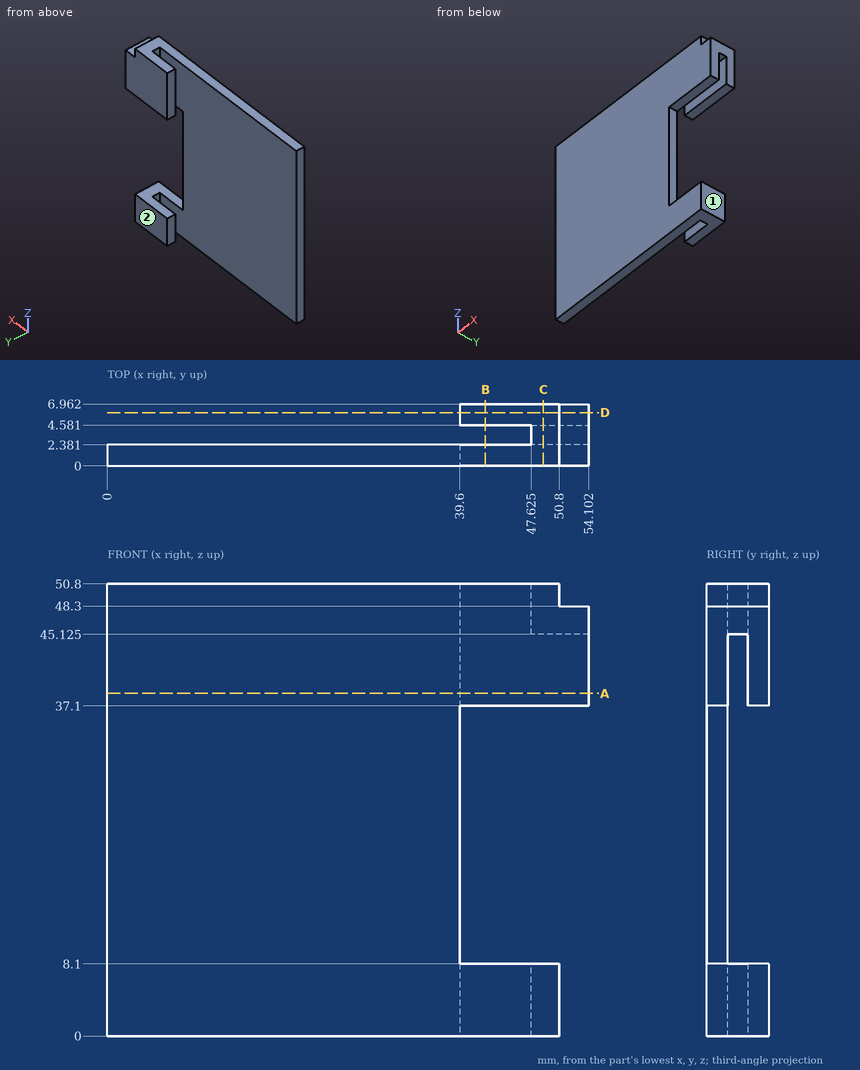
Could you check a few things on this drawing? It's one solid part, dimensions in mm from its lowest x, y, z. A direction names the side the tool comes from. Coordinates: 2 decimals unless noted, no trailing zeros. Write each loop counter-clockwise with the first axis right and the second up, starting at its lowest first coordinate (ties: lowest second). Pieces come first, ordered by that corner, then holes. Notation, with made-up numbers: (60.25, -26.5) - (106.25, -26.5) arc R24 ccw to (106.25, -9.5) - close; hole circle Ø7 at (-16.5, 6). An arc over 180 degrees is marked (long way). Return JSON: item names as keys, results as strings. Group by question number.
Item 1: If we section it at D-D (y = 6): Write out the boundary of the cut face in (x, z), then the cut area to 3 significant figures.
Item 2: If we section it at A-A (z = 38.5): Write out the boundary of the cut face in (x, y).
Item 3: I'm going to push flat-ended pins straight in: pin 1 Ø1.2 at (y, z) = (5.5, 3.5) entering from -X; pin 2 Ø1.2 at (x, y) = (46.5, 1.5) entering from -Z; pin 3 Ø1.1 at (y, z) = (3.5, 4.5) entering from -X (1 decimal); pin 4 Ø1.3 at (y, z) = (2.5, 50) entering from +X. Where does each tip first touch, or does it pass through?
Item 4: If we section it at B-B (x = 42.5): Write out the boundary of the cut face in (y, z), then the cut area to 3 significant figures.
Item 5: If we section it at C-C (x = 49): Write out the boundary of the cut face in (y, z) (1 decimal), then the cut area to 3 significant figures.
Item 6: Which directions (+Z, -Z, +X, -X, +Y, -Y) give clear straight access to the entire face, cutting with the end or side of a thin tool? Please do the marked faces 1 and 2.
Item 7: Please list where these lines run through material, in increasing order: probe 1 along Y at (x, z) = (36.5, 30.5); probe 2 along Z at (x, y) = (43.5, 6.75); probe 3 along Y at (x, z) = (40, 39.5).
Return value:
{
 "1": {"outline": "(39.6, 0) - (50.8, 0) - (50.8, 8.1) - (39.6, 8.1) - close; (39.6, 37.1) - (54.1, 37.1) - (54.1, 48.3) - (50.8, 48.3) - (50.8, 50.8) - (39.6, 50.8) - close", "area": "281 mm^2"},
 "2": {"outline": "(0, 0) - (54.1, 0) - (54.1, 2.38) - (0, 2.38) - close; (39.6, 4.58) - (54.1, 4.58) - (54.1, 6.96) - (39.6, 6.96) - close"},
 "3": {"pin 1": "stops at x = 39.6", "pin 2": "stops at z = 0", "pin 3": "stops at x = 47.6", "pin 4": "stops at x = 50.8"},
 "4": {"outline": "(0, 0) - (2.38, 0) - (2.38, 8.1) - (0, 8.1) - close; (0, 37.1) - (2.38, 37.1) - (2.38, 50.8) - (0, 50.8) - close; (4.58, 0) - (6.96, 0) - (6.96, 8.1) - (4.58, 8.1) - close; (4.58, 37.1) - (6.96, 37.1) - (6.96, 50.8) - (4.58, 50.8) - close", "area": "104 mm^2"},
 "5": {"outline": "(0, 0) - (7, 0) - (7, 8.1) - (0, 8.1) - close; (0, 37.1) - (2.4, 37.1) - (2.4, 45.1) - (4.6, 45.1) - (4.6, 37.1) - (7, 37.1) - (7, 50.8) - (0, 50.8) - close", "area": "134 mm^2"},
 "6": {"face 1": "-Z, +X, +Y, -Y", "face 2": "+Z, -Z, +X, -X, +Y"},
 "7": {"probe 1": "y = 0 to 2.38", "probe 2": "z = 0 to 8.1, 37.1 to 50.8", "probe 3": "y = 0 to 2.38, 4.58 to 6.96"}
}
